Verification items for the finished model (mm, model axes). Coordinates: 2 decimals unless noted, no trailing zeros. Write each loop counter-clockwise with the first axis right and the second up, starting at its lowest first coordinate (ties: lowest second). Pieces come first, ordered by that corner, then holes. Notation, with made-up numbers: (17.5, 61) -> (36.5, 61) arc R36 ccw to (36.5, 98) -> close; hole circle Ø10 at (66.25, 87). An arc over 180 degrees is marked (long way). Write item = value, one per line. Start each with the question number.
(1) Material ranges on probe 1 along Y at (x, z) = (0, 13); probe 2 along Y at (x, z) = (-52, 9.5); probe 3 along Y at (x, z) = (12, 13), recorded low to high. Write a range as [from, to].
(2) Section check B-B (z = 13.5). State how many separate pieces and enclosed holes the cut face has, plus the area to 3 significant figures.
(3) Section check A-A (x = -51). Record the cut outline in (y, z).
(4) Section check C-C (y = 51). Record the cut outline in (x, z), plus the area to 3 significant figures.
(5) Gauge pin test, flat ends, axial feed: pin 1 Ø6.5 at (x, y) = (-163.74, 212.61) entering from -Z; pin 2 Ø10 at (y, z) = (104.5, 5.5) entering from -X; pin 3 Ø2 at (y, z) = (135.5, 15.5) entering from +X. Record the tip position at first contact, or that the pin passes through.
(6) Section check D-D (x = 187). Record the cut outline in (y, z), plus the area to 3 significant figures.
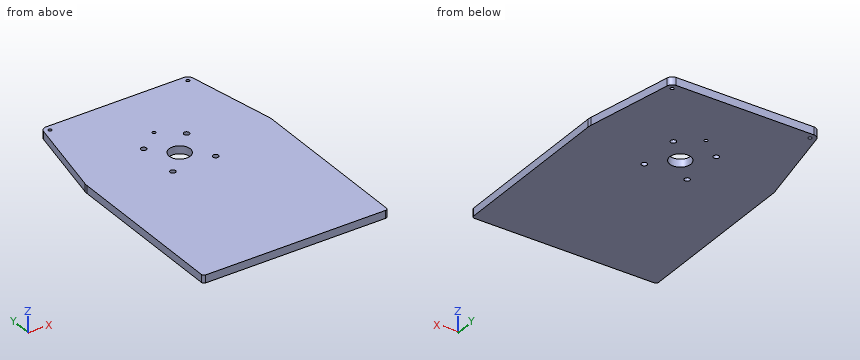
```python
from build123d import *

# Parameters (mm, degrees)
SKETCH_R   = 25
SKETCH_R_2 = 6.5
SKETCH_R_3 = 4.1
PAD_DEPTH  = 18.5


with BuildPart() as part:
    # Sketch → Pad (new body)
    with BuildSketch(Plane.XY):
        with BuildLine():
            Line((-220, 0), (-220, -400))
            ThreePointArc((-220, -400), (-218.242641, -404.242641), (-214, -406))
            Line((-214, -406), (214, -406))
            ThreePointArc((214, -406), (218.242641, -404.242641), (220, -400))
            Line((220, -400), (220, 0))
            ThreePointArc((220, 0), (219.751495, 4.978826), (219.008452, 9.908162))
            Line((219.008452, 9.908162), (177.466268, 215.387043))
            ThreePointArc((177.466268, 215.387043), (172.608438, 223.448808), (163.743902, 226.612757))
            Line((-163.743902, 226.612757), (163.743902, 226.612757))
            ThreePointArc((-163.743902, 226.612757), (-172.608438, 223.448808), (-177.466268, 215.387043))
            Line((-219.008452, 9.908162), (-177.466268, 215.387043))
            ThreePointArc((-219.008452, 9.908162), (-219.751495, 4.978826), (-220, 0))
        make_face()
        Circle(SKETCH_R, mode=Mode.SUBTRACT)
        with Locations((51, 51)):
            Circle(SKETCH_R_2, mode=Mode.SUBTRACT)
        with Locations((-51, 51)):
            Circle(SKETCH_R_2, mode=Mode.SUBTRACT)
        with Locations((-51, -51)):
            Circle(SKETCH_R_2, mode=Mode.SUBTRACT)
        with Locations((51, -51)):
            Circle(SKETCH_R_2, mode=Mode.SUBTRACT)
        with Locations((0, 90)):
            Circle(SKETCH_R_3, mode=Mode.SUBTRACT)
        with Locations((163.743902, 212.612757)):
            Circle(SKETCH_R_3, mode=Mode.SUBTRACT)
        with Locations((-163.743902, 212.612757)):
            Circle(SKETCH_R_3, mode=Mode.SUBTRACT)
    extrude(amount=PAD_DEPTH)


solid = part.part
```
Response:
q1.probe_1 = [-406, -25], [25, 85.9], [94.1, 226.61]
q1.probe_2 = [-406, -57.42], [-44.58, 44.58], [57.42, 226.61]
q1.probe_3 = [-406, -21.93], [21.93, 226.61]
q2.separate_pieces = 1
q2.enclosed_holes = 8
q2.area = 266,000 mm2
q3.outline = (-406, 0) -> (-57.5, 0) -> (-57.5, 18.5) -> (-406, 18.5) -> close; (-44.5, 0) -> (44.5, 0) -> (44.5, 18.5) -> (-44.5, 18.5) -> close; (57.5, 0) -> (226.61, 0) -> (226.61, 18.5) -> (57.5, 18.5) -> close
q4.outline = (-210.7, 0) -> (-57.5, 0) -> (-57.5, 18.5) -> (-210.7, 18.5) -> close; (-44.5, 0) -> (44.5, 0) -> (44.5, 18.5) -> (-44.5, 18.5) -> close; (57.5, 0) -> (210.7, 0) -> (210.7, 18.5) -> (57.5, 18.5) -> close
q4.area = 7,310 mm2
q5.pin_1 = through
q5.pin_2 = -200.9
q5.pin_3 = 193.82
q6.outline = (-406, 0) -> (168.23, 0) -> (168.23, 18.5) -> (-406, 18.5) -> close
q6.area = 10,600 mm2
